Geometry: final body of the model. Coordinates: model frame, mm. A direction names the side the tool comes from. Round coordinates to 2 decimals unless told otherwise and drop trailing zeros. Loops run counter-clockwise (first coordinate to the right, second up) from the corner with the lowest first, then second, coordinate; pieces in that order, holes last. Notation, with made-up numbers: (0, 73.25) -> (29, 73.25) arc R27 cw to (29, 99.25) -> close; hole circle Ø5 at (12.5, 80.5). An arc over 180 degrees is marked (long way). Answer in a Markdown table with one row per item.
```python
from build123d import *

# Parameters (mm, degrees)
F1_DEPTH = 12.7
F2_SIZE  = 5.08
F3_R     = 5.08


with BuildPart() as f1:
    # F0 (on Top) → F1 (new body)
    with BuildSketch(Plane.XY):
        Polygon((22.117395, 32.115713), (68.473089, 89.075649), (-30.903824, 9.998288), (-4.847682, 9.998288), (-43.931895, -29.388905), (-17.875753, -29.388905), (-68.473148, -89.075649), (33.630579, -8.180417), (5.150606, -8.180417), (46.355669, 32.115713), align=None)
    extrude(amount=F1_DEPTH)

    # F2
    f2_edges = [f1.edges().sort_by_distance(p)[0] for p in [
        (34.236532, 32.115713, 12.7),
        (45.295242, 60.595681, 12.7),
        (18.784632, 49.536968, 12.7),
        (-17.875753, 9.998288, 12.7),
        (-24.389789, -9.695309, 12.7),
        (-30.903824, -29.388905, 12.7),
        (-43.174451, -59.232277, 12.7),
        (-17.421285, -48.628033, 12.7),
        (19.390592, -8.180417, 12.7),
        (25.753137, 11.967648, 12.7),
    ]]
    chamfer(f2_edges, length=F2_SIZE)

    # F3
    f3_edges = [f1.edges().sort_by_distance(p)[0] for p in [
        (34.236532, 32.115713, 0),
        (45.295242, 60.595681, 0),
        (18.784632, 49.536968, 0),
        (-17.875753, 9.998288, 0),
        (-24.389789, -9.695309, 0),
        (-30.903824, -29.388905, 0),
        (-43.174451, -59.232277, 0),
        (-17.421285, -48.628033, 0),
        (19.390592, -8.180417, 0),
        (25.753137, 11.967648, 0),
    ]]
    fillet(f3_edges, radius=F3_R)


solid = f1.part
```
Item 1: Set-up query: faces 1 (the flat face through (44.971, 60.197, 6.332)), 2 (the flat face through (29.139, 29.54, 10.196)), 3 (the cylindrical face through (20.582, 9.047, 1.449)), 4 (the flat face through (-25.68, -26.81, 10.2)), 5 (the cylindrical face through (-25.16, -27.86, 1.45)). Return all of +Z, -Z, +X, -X, +Y, -Y with unobstructed straight access to the full face (end or side cutting, diameter ignored); none if empty.
Ans:
| item | result |
|---|---|
| face 1 | +Z, -Z, +X |
| face 2 | +Z, +X |
| face 3 | -Z, +X |
| face 4 | +Z, -X |
| face 5 | -Z, -X |
Item 2: Section query A-A, the plane z = 2.75. Output: boundary loops of the cut face in (x, y).
Ans:
| item | result |
|---|---|
| outline | (-64.35, -85.09) -> (32.01, -8.75) -> (3.76, -8.75) -> (44.97, 31.55) -> (20.93, 31.55) -> (64.73, 85.38) -> (-29.28, 10.56) -> (-3.49, 10.56) -> (-42.57, -28.82) -> (-16.65, -28.82) -> close |
Item 3: Ray query, L1, parallel to Y at x = -18.5, z = 8; L2, parallel to Y at x = 23.5, z = 8.25; L3, parallel to Y at x = 11.5, z = 11.25. Return the intervals inside material, ascending.
Ans:
| item | result |
|---|---|
| L1 | -49 to -30.71, -29.01 to -4.3, 10.38 to 19.38 |
| L2 | -15.4 to -8.81, 10.65 to 31.49, 34.81 to 52.48 |
| L3 | -21.08 to -11.81, 3.11 to 39.1 |
Item 4: Section query B-B, the plane x = -28. State how many separate pieces and enclosed holes the cut face has, and give its area (3 significant figures).
Ans:
| item | result |
|---|---|
| separate pieces | 3 |
| enclosed holes | 0 |
| area | 318 mm2 |
Item 5: First-contact query: P1, Ø2, axis at x = 9.5, z = 5.5, coming from the +Y side; P2, Ø1.5, axis at y = -65, z = 7, coming from the +X side; P3, Ø0.8, axis at x = 31, z = 6.5, coming from the +Y side. Flat tips, straight axial feed; report the tip coordinate or a pass-through.
Ans:
| item | result |
|---|---|
| P1 | y = 42.94 |
| P2 | x = -37.14 |
| P3 | y = 59.58 |
Item 6: Mould query, pull axis Y, two halves, no side actions, for faces 6 (the flat face through (-12.045, 12.574, 10.196)), 7 (the flat face through (-18.136, -49.194, 6.332)), 8 (the cylindrical face through (19.04, 47.79, 1.45)), 9 (the flat face through (-24.116, -9.42, 6.332)). Classes: released by +Y, released by -Y, zero draft, split by the parting line, or undercut.
Ans:
| item | result |
|---|---|
| face 6 | undercut |
| face 7 | released by -Y |
| face 8 | released by +Y |
| face 9 | undercut |
